Job drawing, mm, ordinate dimensions from the low corner. One solid piece. A direction names the side the tool comes from. Give positions to 0.01 mm unless a question says otherwise; leave off trailing zeros. Loops run counter-clockwise (first coordinate to the right, second up) from the corner with the lowest first, then second, coordinate; pieces in that order, holes last. Notation, with made-up numbers: M 57,32.25 L 88,32.25 A20 ccw 88,44.25 Z; hole C -17.5,23.25 d5. An arc over 180 degrees is marked long. Answer in a Markdown table with one row per item.
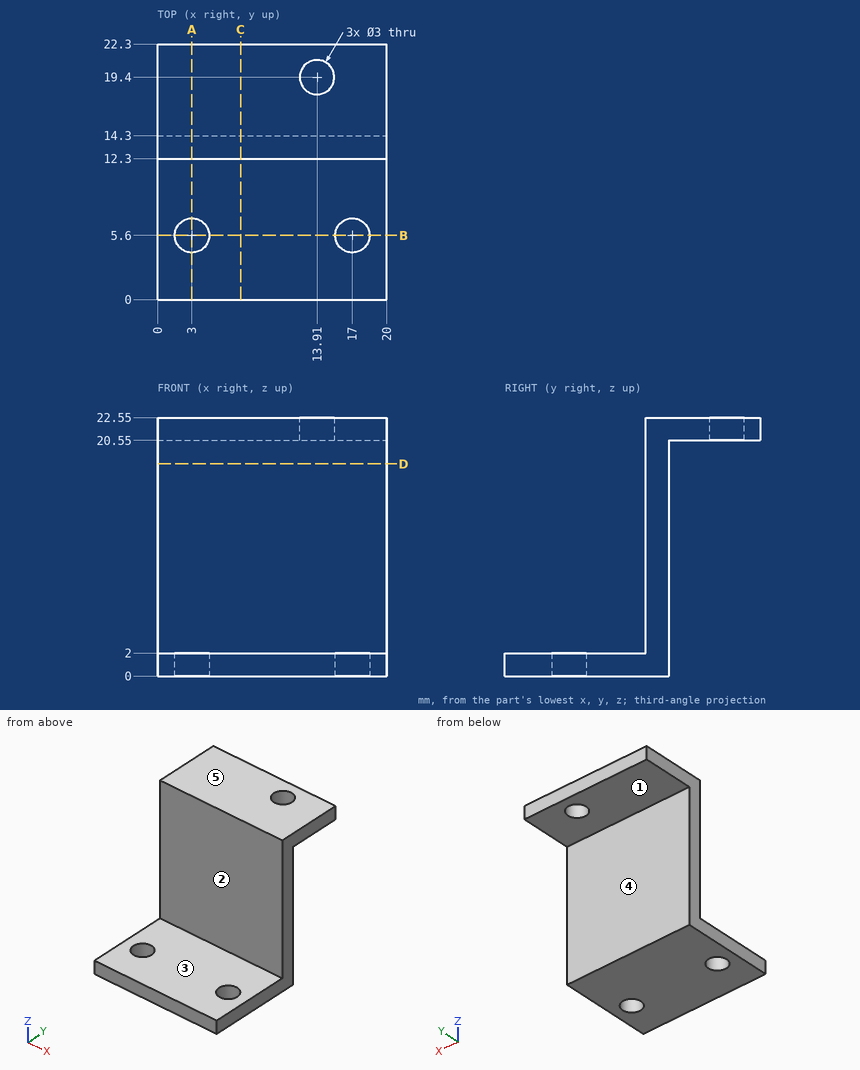
(1) Pin check, flat tips, straight feed: pin 1 Ø1.5 at (x, z) = (16, 8) entering from +Y; pin 2 Ø3.5 at (x, y) = (3, 5.6) entering from +Z; pin 3 Ø10 at (x, z) = (11, 10) entering from -Y. Stop position of each tip, or through.
Recorded:
| item | result |
|---|---|
| pin 1 | stops at y = 14.3 |
| pin 2 | stops at z = 2 |
| pin 3 | stops at y = 12.3 |
(2) Pull direction Z, two halves, no side cores. Call the marked faces 1, 2 and 3: +Z half, -Z half, draft (parallel to the pull), parting line (faces both ways), or undercut.
Recorded:
| item | result |
|---|---|
| face 1 | -Z half |
| face 2 | draft |
| face 3 | +Z half |
(3) Saw through at D-D (z = 18.5). Write the cut outline in (x, y).
Recorded:
| item | result |
|---|---|
| outline | M 0,12.3 L 20,12.3 L 20,14.3 L 0,14.3 Z |
(4) Saw through at A-A (x = 3). Write the cut outline in (y, z).
Recorded:
| item | result |
|---|---|
| outline | M 0,0 L 4.1,0 L 4.1,2 L 0,2 Z; M 7.1,0 L 14.3,0 L 14.3,20.55 L 22.3,20.55 L 22.3,22.55 L 12.3,22.55 L 12.3,2 L 7.1,2 Z |
(5) Drill centre lines: line 1 along Y through (x, z) = (3, 1.65); line 2 along Y through (x, z) = (5.25, 4); line 3 along Y through (x, z) = (13.91, 22.05). Where is each one in solid material? Low to high.
Recorded:
| item | result |
|---|---|
| line 1 | y = 0 to 4.1, 7.1 to 14.3 |
| line 2 | y = 12.3 to 14.3 |
| line 3 | y = 12.3 to 17.9, 20.9 to 22.3 |
(6) Which spindle directions (+Z, -Z, +X, -X, +Y, -Y) get a long thin tool onto all of the face, cutting with end or side? Do the marked faces 4 and 5. Say none if no direction does.
Recorded:
| item | result |
|---|---|
| face 4 | -Z, +X, -X, +Y |
| face 5 | +Z, +X, -X, +Y, -Y |
(7) Saw through at B-B (y = 5.6). Write the cut outline in (x, z), plus the area to 3 significant figures.
Recorded:
| item | result |
|---|---|
| outline | M 0,0 L 1.5,0 L 1.5,2 L 0,2 Z; M 4.5,0 L 15.5,0 L 15.5,2 L 4.5,2 Z; M 18.5,0 L 20,0 L 20,2 L 18.5,2 Z |
| area | 28.0 mm^2 |
(8) Saw through at C-C (x = 7.25). Write the cut outline in (y, z).
Recorded:
| item | result |
|---|---|
| outline | M 0,0 L 14.3,0 L 14.3,20.55 L 22.3,20.55 L 22.3,22.55 L 12.3,22.55 L 12.3,2 L 0,2 Z |
